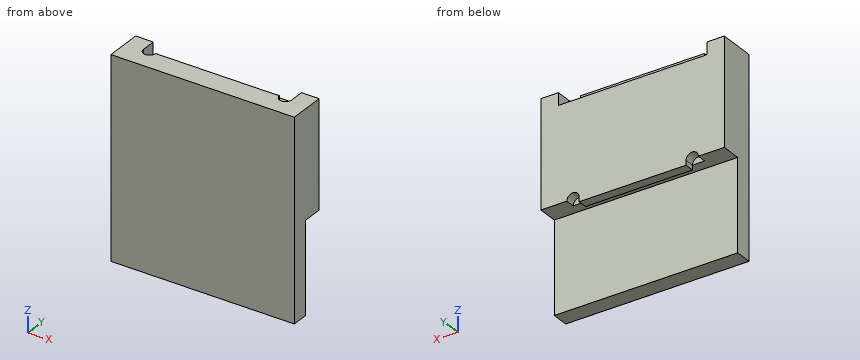
```python
from build123d import *

# Parameters (mm, degrees)
F0_W      = 120
F0_H      = 24
F1_DEPTH  = 130
F2_W      = 97
F2_H      = 9.5
F3_DEPTH  = 8
F5_DEPTH  = 8
F7_DEPTH  = 120.001
F8_W      = 25
F8_H      = 3
F9_DEPTH  = 13
F11_DEPTH = 6.2


with BuildPart() as f1:
    # F0 (on Top) → F1 (new body)
    with BuildSketch(Plane.XY):
        Rectangle(F0_W, F0_H)
    extrude(amount=F1_DEPTH)

    # F2 (on face) → F3 (cut)
    with BuildSketch(Plane.XY.offset(130)):
        with Locations((0, 7.25)):
            Rectangle(F2_W, F2_H)
    extrude(amount=-F3_DEPTH, mode=Mode.SUBTRACT)

    # F4 (on face) → F5 (cut, through all)
    with BuildSketch(Plane.XY.offset(130)):
        with BuildLine():
            Line((-40.5, 2.5), (-48.5, 2.5))
            ThreePointArc((-48.5, 2.5), (-44.5, -1.5), (-40.5, 2.5))
        make_face()
        with BuildLine():
            ThreePointArc((40.5, 2.5), (44.5, -1.5), (48.5, 2.5))
            Line((48.5, 2.5), (40.5, 2.5))
        make_face()
    extrude(amount=-F5_DEPTH, mode=Mode.SUBTRACT)

    # F6 (on face) → F7 (cut, through all)
    with BuildSketch(Plane.YZ.offset(60)):
        Polygon((-1, 0), (12, 0), (12, 57), (5.8, 57), (5.8, 60), (-1, 60), align=None)
    extrude(amount=-F7_DEPTH, mode=Mode.SUBTRACT)

    # F8 (on face) → F9 (cut, through all)
    with BuildSketch(Plane(origin=(0, 12, 0), x_dir=(-1, 0, 0), z_dir=(0, 1, 0))):
        with Locations((-47.5, 58.5)):
            Rectangle(F8_W, F8_H)
        with Locations((47.5, 58.5)):
            Rectangle(F8_W, F8_H)
    extrude(amount=-F9_DEPTH, mode=Mode.SUBTRACT)

    # F10 (on face) → F11 (cut, through all)
    with BuildSketch(Plane(origin=(0, 12, 0), x_dir=(-1, 0, 0), z_dir=(0, 1, 0))):
        with BuildLine():
            Line((-43, 60), (-35, 60))
            ThreePointArc((-35, 60), (-39, 64), (-43, 60))
        make_face()
        with BuildLine():
            ThreePointArc((43, 60), (39, 64), (35, 60))
            Line((35, 60), (43, 60))
        make_face()
    extrude(amount=-F11_DEPTH, mode=Mode.SUBTRACT)


solid = f1.part
```
The model under review builds one solid part; all positions refer to its coordinate system, in mm. Round coordinates to 2 decimals unless told otherwise and drop trailing zeros. Loops run counter-clockwise (first coordinate to the right, second up) from the corner with the lowest first, then second, coordinate; pieces in that order, holes last. Notation, with made-up numbers: (0.5, 80.5) - (42.5, 80.5) arc R16 cw to (42.5, 100.5) - close; hole circle Ø8 at (13.25, 71.25). An arc over 180 degrees is marked (long way). Use a Markdown table: item, result. Add a question column.
Q1. Add section C-C (z = 38). State the section outline as (x, y) points, plus the area to 3 significant figures.
Q2. For probe 1 along Y at (x, z) = (-54, 14.5); probe 2 along Z at (x, y) = (24, 1); probe 3 along Z at (x, y) = (-19, 7.25), list the stretches that pass through material, from the lowest coordinate up.
Q3. Add section B-B (y = 9.5). State the section outline as (x, z) points.
Q4. Add section A-A (x = 39). State the section outline as (y, z) points, plus the area to 3 significant figures.
Q5. Add section D-D (x = -19). State the section outline as (y, z) points, plus the area to 3 significant figures.
Q6. Insertion check: pin 1 Ø1.9 at (x, y) = (0.5, 8) entering from -Z; pin 2 Ø0.9 at (y, z) = (9, 59) entering from +X; pin 3 Ø1.5 at (x, y) = (-21.5, 7) entering from +Z; pin 4 Ø4.5 at (x, z) = (37, 62.5) entering from +Y. Each pin has a flat end and moves straight along its axis. Give the tip position at first contact, or say it passes through.
Worked answers:
| question | item | result |
|---|---|---|
| 1 | outline | (-60, -12) - (60, -12) - (60, -1) - (-60, -1) - close |
| 1 | area | 1,320 mm² |
| 2 | probe 1 | -12 to -1 |
| 2 | probe 2 | 60 to 130 |
| 2 | probe 3 | 57 to 122 |
| 3 | outline | (-60, 60) - (-43, 60) arc R4 cw to (-35, 60) - (-35, 57) - (35, 57) - (35, 60) arc R4 cw to (43, 60) - (60, 60) - (60, 130) - (48.5, 130) - (48.5, 122) - (-48.5, 122) - (-48.5, 130) - (-60, 130) - close |
| 4 | outline | (-12, 0) - (-1, 0) - (-1, 60) - (5.8, 60) - (5.8, 64) - (12, 64) - (12, 122) - (2.5, 122) - (2.5, 130) - (-12, 130) - close |
| 4 | area | 2,240 mm² |
| 5 | outline | (-12, 0) - (-1, 0) - (-1, 60) - (5.8, 60) - (5.8, 57) - (12, 57) - (12, 122) - (2.5, 122) - (2.5, 130) - (-12, 130) - close |
| 5 | area | 2,280 mm² |
| 6 | pin 1 | z = 57 |
| 6 | pin 2 | x = 35 |
| 6 | pin 3 | z = 122 |
| 6 | pin 4 | y = 12 |
